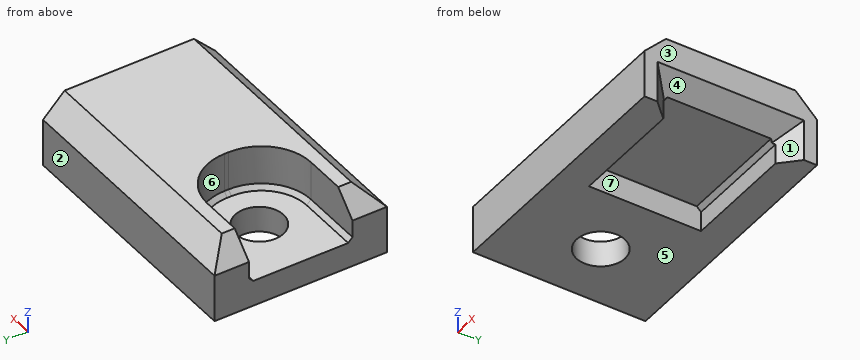
Autodesk Inventor part; units mm, degrees
ref_plane "YZ Plane" through (0, 0, 0) normal (1, 0, 0) x (0, 1, 0)
ref_plane "XZ Plane" through (0, 0, 0) normal (0, 1, 0) x (-1, 0, 0)
ref_plane "XY Plane" through (0, 0, 0) normal (0, 0, 1) x (1, 0, 0)
sketch "Sketch1" plane through (0, 0, 0) normal (0, 0, 1) x (1, 0, 0)
  line L0 (-15, -10) -> (15, -10)
  line L1 (15, -10) -> (15, 10)
  line L2 (15, 10) -> (-15, 10)
  line L3 (-15, 10) -> (-15, -10)
  line L4 (-15, -10) -> (15, 10) construction
  line L5 (15, -10) -> (-15, 10) construction
  point P0 (0, 0)
  dimension "d0" = 20
  dimension "d1" = 30
extrude "Extrusion1" add sketch "Sketch1" along normal blind 8
sketch "Sketch2" plane through (15, -10, 0) normal (1, 0, 0) x (0, 0, -1)
  line L0 (-9.6, 10) -> (1.6, 10)
  line L1 (0, 0) -> (0, 20)
  line L2 (0, 3.5) -> (-2.8, 3.5)
  line L3 (-2.8, 3.5) -> (-2.8, 16.5)
  line L4 (-2.8, 16.5) -> (0, 16.5)
  line L5 (0, 16.5) -> (0, 3.5)
  point P0 (0, 10)
  point P1 (0, 16.5)
  dimension "d4" = 2.8
  dimension "d5" = 13
  dimension "d6" = 6.5
extrude "Extrusion2" cut sketch "Sketch2" against normal blind 15
chamfer "Chamfer1" distance 2 angle 45 3 edges at (15, 0, 2.8) (15, 6.5, 1.4) (15, -6.5, 1.4)
chamfer "Chamfer2" distance 0.5 angle 45 2 edges at (6.5, 6.5, 2.8) (6.5, -6.5, 2.8)
sketch "Sketch3" plane through (0, 0, 8) normal (0, 0, 1) x (1, 0, 0)
  line L0 (-21, 0) -> (21, 0)
  line L1 (-2, -6) -> (-15, -6)
  line L2 (-15, -6) -> (-15, 6)
  line L3 (-15, 6) -> (-2, 6)
  line L4 (-2, 6) -> (-2, -6)
  line L5 (-2, -6) -> (-15, 6) construction
  line L6 (-15, -6) -> (-2, 6) construction
  line L7 (-15, 10) -> (-15, -10)
  line L8 (0, -6) -> (0, 6)
  point P0 (0, 0)
  point P1 (-8.5, 0)
  dimension "d15" = 2
  dimension "d16" = 12
extrude "Extrusion3" cut sketch "Sketch3" against normal blind 5
chamfer "Chamfer3" distance 2.5 angle 45 2 edges at (0, 10, 8) (0, -10, 8)
fillet "Fillet1" radius 5.75 2 edges at (-2, 6, 5.5) (-2, -6, 5.5)
chamfer "Chamfer4" distance 2.5 angle 45 2 edges at (-15, -6.75, 8) (-15, 6.75, 8)
sketch "Sketch4" plane through (0, 0, 3) normal (0, 0, 1) x (1, 0, 0)
  line L0 (-21, 0) -> (21, 0)
  circle A0 centre (-7.75, 0) radius 2.8
  arc A1 (-2, 0.25) -> (-7.75, 6) centre (-7.75, 0.25) ccw
  line L1 (-7.75, -6) -> (-15, -6)
  line L2 (-7.75, 6) -> (-7.75, -6) construction
  point P0 (0, 0)
  dimension "d26" = 5.6
  dimension "d27" = 0
extrude "Extrusion4" cut sketch "Sketch4" against normal blind 5
chamfer "Chamfer5" distance 0.5 angle 45 5 edges at (-3.6841, 4.3159, 3) (-11.375, 6, 3) (-2, 0, 3) (-3.6841, -4.3159, 3) (-11.375, -6, 3)
equation "\"d6\" = 0.5 * d5"
properties part number "BatteryHolderFixture_3DPrint"
CAD build for the part. Positions are in the model's coordinates, mm. Face numbers are marked on the shaded views. A direction names the side the tool comes from. Coordinates: 2 decimals unless noted, no trailing zeros. Write each loop counter-clockwise with the first axis right and the second up, starting at its lowest first coordinate (ties: lowest second). Pieces come first, ordered by that corner, then holes. Notation, with made-up numbers: (-39, -39) - (-10, -39) arc R6 ccw to (-10, -34) - close; hole circle Ø6 at (21, 39.5). An arc over 180 degrees is marked (long way). Use a Markdown table: item, result. Add a question column.
Item 1: Mould opens along Y. For the marked faces 1, 2, 3 and 4 say: pulls with the +Y half, pulls with the -Y half, needs draft (parallel to the pull), parting line crosses it, or undercut.
Item 2: Band-saw the part on B-B, the plane x = 2.75. Give the cut face in (y, z).
Item 3: Band-saw the part on C-C, the plane z = 4.5. Give the cut face in (x, y).
Item 4: 3-axis set-ups, long thin cutter, end or side, ignore diameter. For the marked faces 5, 6 and 7: which of +Z, -Z, +X, -X, +Y, -Y reach the whole face in a straight line?
Item 5: Band-saw the part on A-A, the plane z = 0.5. Give the cut face in (x, y), and give its area (3 significant figures).
Item 6: Drill centre lines: L1, parallel to X at y = 0, z = 2.3; L2, parallel to Y at x = -7.75, z = 0.95; L3, parallel to Y at x = 6.75, z = 0.75. Where is each one in solid material? Low to high. Write a range as from..to.
Item 7: Flat gauge pins, fed straight in: pin 1 (2 mm diameter, centred on y = 2, z = 1.5, fed in from +X); pin 2 (7.5 mm diameter, centred on x = -7.75, y = 0, fed in from +Z); pin 3 (2 mm diameter, centred on x = 3.5, y = -1.5, fed in from -Z). Where does each tip first touch, or does it go through?
Numbers:
| question | item | result |
|---|---|---|
| 1 | face 1 | undercut |
| 1 | face 2 | pulls with the +Y half |
| 1 | face 3 | needs draft |
| 1 | face 4 | undercut |
| 2 | outline | (-10, 0) - (-6.5, 0) - (-6.5, 2.3) - (-6, 2.8) - (6, 2.8) - (6.5, 2.3) - (6.5, 0) - (10, 0) - (10, 5.5) - (7.5, 8) - (-7.5, 8) - (-10, 5.5) - close |
| 3 | outline | (-15, -10) - (15, -10) - (15, -8.5) - (14.7, -8.2) - (14.7, 8.2) - (15, 8.5) - (15, 10) - (-15, 10) - (-15, 6) - (-7.75, 6) arc R5.75 cw to (-2, 0.25) - (-2, -0.25) arc R5.75 cw to (-7.75, -6) - (-15, -6) - close |
| 4 | face 5 | -Z, +X, -X, +Y, -Y |
| 4 | face 6 | +Z, -X |
| 4 | face 7 | -Z, +X |
| 5 | outline | (-15, -10) - (15, -10) - (15, -8.5) - (13, -6.5) - (0, -6.5) - (0, 6.5) - (13, 6.5) - (15, 8.5) - (15, 10) - (-15, 10) - close; hole circle Ø5.6 at (-7.75, 0) |
| 5 | area | 376 mm2 |
| 6 | L1 | -15..-10.55, -4.95..0 |
| 6 | L2 | -10..-2.8, 2.8..10 |
| 6 | L3 | -10..-6.5, 6.5..10 |
| 7 | pin 1 | x = 0 |
| 7 | pin 2 | z = 3 |
| 7 | pin 3 | z = 2.8 |
